Part model, mm, in its own coordinate system. Coordinates: 2 decimals unless noted, no trailing zeros. Write each loop counter-clockwise with the first axis right and the second up, starting at its lowest first coordinate (ties: lowest second). Pieces come first, ordered by that corner, then holes. Notation, with made-up numbers: (55.25, 69) -> (71.25, 69) arc R27 cw to (71.25, 94) -> close; hole circle Ø11 at (18.5, -21). An arc over 180 degrees is marked (long way). Write item = value, one per line.
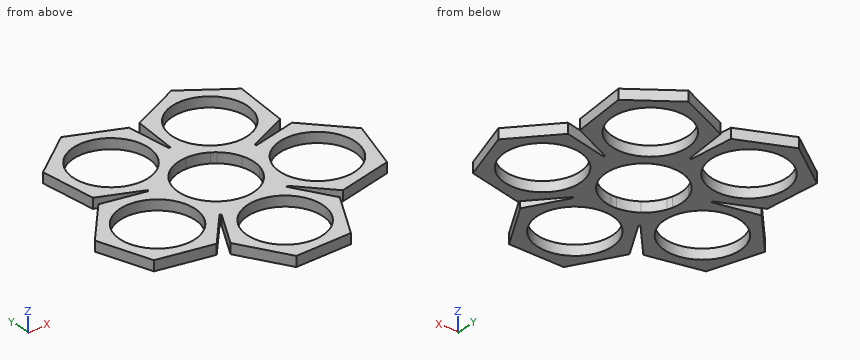
from build123d import *

# Parameters (mm, degrees)
F0_R     = 11
F1_DEPTH = 3


with BuildPart() as f1:
    # F0 (on Top) → F1 (new body)
    with BuildSketch(Plane.XY):
        Polygon((9.692502, -13.691952), (9.947785, -13.691952), (10.0425, -13.400449), (18.702897, -23.105726), (34.559387, -19.809369), (39.632903, -4.429067), (28.849928, 7.654877), (16.016968, 4.987071), (16.095854, 5.22986), (15.847887, 5.410019), (27.754365, 10.64745), (29.519267, 26.746499), (16.459534, 36.324473), (1.634898, 29.803399), (0.206528, 16.774131), (0, 16.924183), (-0.247967, 16.744024), (-1.549757, 29.686213), (-16.315477, 36.339614), (-29.460351, 26.878826), (-27.839506, 10.764637), (-15.889326, 5.379912), (-16.095854, 5.22986), (-16.001139, 4.938357), (-28.712167, 7.699638), (-39.602786, -4.287382), (-34.667032, -19.712445), (-18.840659, -23.150488), (-10.026672, -13.449163), (-9.947785, -13.691952), (-9.641281, -13.691952), (-16.195339, -24.927575), (-8.160391, -38.989362), (8.034947, -39.061787), (16.195339, -25.072425), align=None)
        with Locations((0, -25)):
            Circle(F0_R, mode=Mode.SUBTRACT)
        with Locations((-23.776413, -7.725425)):
            Circle(F0_R, mode=Mode.SUBTRACT)
        with Locations((23.776413, -7.725425)):
            Circle(F0_R, mode=Mode.SUBTRACT)
        with BuildLine():
            ThreePointArc((-0.804417, -10.970548), (-3.77969, -10.330244), (-6.465638, -8.899187))
            ThreePointArc((-6.465638, -8.899187), (-8.686922, -6.74814), (-10.221788, -4.063872))
            ThreePointArc((-10.221788, -4.063872), (-10.476718, -3.352369), (-10.682189, -2.62504))
            ThreePointArc((-10.682189, -2.62504), (-10.992634, 0.402478), (-10.461622, 3.399187))
            ThreePointArc((-10.461622, 3.399187), (-9.102269, 6.176464), (-7.023678, 8.465692))
            ThreePointArc((-7.023678, 8.465692), (-6.425776, 8.928012), (-5.797539, 9.348184))
            ThreePointArc((-5.797539, 9.348184), (-3.014132, 10.578989), (0, 11))
            ThreePointArc((0, 11), (3.06141, 10.565404), (5.880916, 9.295958))
            ThreePointArc((5.880916, 9.295958), (6.50537, 8.870184), (7.099113, 8.402535))
            ThreePointArc((7.099113, 8.402535), (9.129799, 6.135697), (10.461622, 3.399187))
            ThreePointArc((10.461622, 3.399187), (10.994324, 0.353315), (10.658284, -2.720474))
            ThreePointArc((10.658284, -2.720474), (10.446316, -3.445937), (10.185032, -4.155131))
            ThreePointArc((10.185032, -4.155131), (8.656658, -6.78692), (6.465638, -8.899187))
            ThreePointArc((6.465638, -8.899187), (3.733456, -10.347043), (0.706266, -10.977303))
            ThreePointArc((0.706266, -10.977303), (-0.049191, -10.99989), (-0.804417, -10.970548))
        make_face(mode=Mode.SUBTRACT)
        with Locations((-14.694631, 20.225425)):
            Circle(F0_R, mode=Mode.SUBTRACT)
        with Locations((14.694631, 20.225425)):
            Circle(F0_R, mode=Mode.SUBTRACT)
    extrude(amount=F1_DEPTH)


solid = f1.part
Q1. Saw through at A-A on x = 32. Give the cut face in (y, z), and give its area (3 significant figures).
Model answer:
outline = (-20.34, 0) -> (-15.03, 0) -> (-15.03, 3) -> (-20.34, 3) -> close; (-0.42, 0) -> (4.12, 0) -> (4.12, 3) -> (-0.42, 3) -> close
area = 29.6 mm²
Q2. Saw through at B-B on y = -33. Give the cut face in (x, z), and give its area (3 significant figures).
Model answer:
outline = (-11.58, 0) -> (-7.55, 0) -> (-7.55, 3) -> (-11.58, 3) -> close; (7.55, 0) -> (11.57, 0) -> (11.57, 3) -> (7.55, 3) -> close
area = 24.2 mm²
Q3. Pin check, flat tip, straight feed: pin 1 (1.5 mm diameter, centred on y = -24, z = 2.5, fed in from +X). Stop position of the tip, or through.
Model answer:
pin_1 = 16.01
Q4. Saw through at C-C on y = 14.5. Give the cut face in (x, z), and give its area (3 significant figures).
Model answer:
outline = (-28.22, 0) -> (-24.09, 0) -> (-24.09, 3) -> (-28.22, 3) -> close; (-5.3, 0) -> (5.3, 0) -> (5.3, 3) -> (-5.3, 3) -> close; (24.09, 0) -> (28.18, 0) -> (28.18, 3) -> (24.09, 3) -> close
area = 56.5 mm²
Q5. Saw through at D-D on x = 23. Give the cut face in (y, z).
Model answer:
outline = (-22.21, 0) -> (-18.7, 0) -> (-18.7, 3) -> (-22.21, 3) -> close; (3.25, 0) -> (6.44, 0) -> (6.44, 3) -> (3.25, 3) -> close; (8.56, 0) -> (13.01, 0) -> (13.01, 3) -> (8.56, 3) -> close; (27.44, 0) -> (31.53, 0) -> (31.53, 3) -> (27.44, 3) -> close
Q6. Probe line 1 (Y direction, x = 7.5, z = 2); line 2 (Y direction, x = -12, z = 1.25); line 3 (Y direction, x = 23, z = 0.7). List the from-to ranges inside material, lowest first. Write a range as from..to.
Model answer:
line_1 = -39.06..-33.05, -16.95..-8.05, 8.05..11.9, 28.55..32.38
line_2 = -32.27..-17.74, -15.62..9.56, 30.89..34.4
line_3 = -22.21..-18.7, 3.25..6.44, 8.56..13.01, 27.44..31.53
